Check sheet for the modelled part. Datum: model origin and axes. Units: mm. Coordinates: 2 decimals unless noted, no trailing zeros. Loops run counter-clockwise (first coordinate to the right, second up) from the corner with the lowest first, then second, coordinate; pieces in that order, holes last. Notation, with made-up numbers: M 42,-12.5 L 55,-12.5 A21 ccw 55,20.5 Z; hole C 52,-10.5 d1. An arc over 180 degrees is marked long. Answer as CSV lines item,"result". Start each with the question number.
from build123d import *

# Parameters (mm, degrees)
BASE_FLANGE1_DEPTH   = 3.03784
M8_CLEARANCE_HOLE1_D = 9


# Sheet-metal steps are written as plain solids
with BuildPart() as part:
    # Sketch1 → Base-Flange1 (new body)
    with BuildSketch(Plane(origin=(0, 0, 0), x_dir=(0, 0, -1), z_dir=(1, 0, 0))):
        with BuildLine():
            Line((-107.95, -152.4), (-222.25, -152.4))
            ThreePointArc((-222.25, -152.4), (-226.740128061, -150.540128061), (-228.6, -146.05))
            Line((-228.6, -146.05), (-228.6, 146.05))
            ThreePointArc((-228.6, 146.05), (-226.740128061, 150.540128061), (-222.25, 152.4))
            Line((-222.25, 152.4), (222.25, 152.4))
            ThreePointArc((222.25, 152.4), (226.740128061, 150.540128061), (228.6, 146.05))
            Line((228.6, 146.05), (228.6, -146.05))
            ThreePointArc((228.6, -146.05), (226.740128061, -150.540128061), (222.25, -152.4))
            Line((222.25, -152.4), (6.35, -152.4))
            ThreePointArc((6.35, -152.4), (1.859871939, -150.540128061), (0, -146.05))
            Line((0, -146.05), (0, -95.25))
            ThreePointArc((0, -95.25), (-1.859871939, -90.759871939), (-6.35, -88.9))
            Line((-6.35, -88.9), (-95.25, -88.9))
            ThreePointArc((-95.25, -88.9), (-99.740128061, -90.759871939), (-101.6, -95.25))
            Line((-101.6, -95.25), (-101.6, -146.05))
            ThreePointArc((-101.6, -146.05), (-103.459871939, -150.540128061), (-107.95, -152.4))
        make_face()
    extrude(amount=-BASE_FLANGE1_DEPTH)

    # M8 Clearance Hole1 (through all)
    with Locations(Plane(origin=(0, 0, 0), x_dir=(0, 0, -1), z_dir=(1, 0, 0))):
        with Locations((-209.55, 101.6), (-209.55, -101.6), (209.55, -101.6), (209.55, 101.6)):
            Hole(M8_CLEARANCE_HOLE1_D / 2)


solid = part.part
Item 1: Sectioned sample at B-B, the plane z = -209.55. Record the boundary of the cut face in (x, y), and give its area (3 significant figures).
Item 2: Sectioned sample at A-A, the plane y = 101.6. Record the boundary of the cut face in (x, z), and give its area (3 significant figures).
Item 3: Sectioned sample at D-D, the plane z = 88. Record the boundary of the cut face in (x, y).
Item 4: Release check for a two-part mould opening along Y. For faces 1 (the face through (-1.54, 99.88, -205.39)), 2 (the face through (-3.038, 2, -3)) record: released by +Y, released by -Y, zero draft, split by the parting line, or undercut.
Item 5: Sectioned sample at C-C, the plane x = -2.2. Record the boundary of the cut face in (y, z).
Item 6: Go/stop test with a flat-tipped pin: pin 1 (7 mm diameter, centred on y = 101.6, z = 209.55, fed in from -X) (3 decimals). Record where the tip stops, or that it passes through.
Item 7: Material ranges on line 1 (Y direction, x = -2.4, z = -209.55); line 2 (Z direction, x = -1.4, y = -105); line 3 (Y direction, x = -2.8, z = 19.5), recorded low to high. Write a range as from..to.
Reply:
1,outline,"M -3.04,-152.4 L 0,-152.4 L 0,-106.1 L -3.04,-106.1 Z; M -3.04,-97.1 L 0,-97.1 L 0,97.1 L -3.04,97.1 Z; M -3.04,106.1 L 0,106.1 L 0,152.4 L -3.04,152.4 Z"
1,area,"871 mm²"
2,outline,"M -3.04,-228.6 L 0,-228.6 L 0,-214.05 L -3.04,-214.05 Z; M -3.04,-205.05 L 0,-205.05 L 0,205.05 L -3.04,205.05 Z; M -3.04,214.05 L 0,214.05 L 0,228.6 L -3.04,228.6 Z"
2,area,"1,330 mm²"
3,outline,"M -3.04,-88.9 L 0,-88.9 L 0,152.4 L -3.04,152.4 Z"
4,face 1,"undercut"
4,face 2,"zero draft"
5,outline,"M -152.4,-222.25 A6.35 ccw -146.05,-228.6 L 146.05,-228.6 A6.35 ccw 152.4,-222.25 L 152.4,222.25 A6.35 ccw 146.05,228.6 L -146.05,228.6 A6.35 ccw -152.4,222.25 L -152.4,107.95 A6.35 ccw -146.05,101.6 L -95.25,101.6 A6.35 cw -88.9,95.25 L -88.9,6.35 A6.35 cw -95.25,0 L -146.05,0 A6.35 ccw -152.4,-6.35 Z; hole C -101.6,-209.55 d9; hole C -101.6,209.55 d9; hole C 101.6,-209.55 d9; hole C 101.6,209.55 d9"
6,pin 1,"through"
7,line 1,"-152.4..-106.1, -97.1..97.1, 106.1..152.4"
7,line 2,"-228.6..-212.5, -206.6..0, 101.6..206.6, 212.5..228.6"
7,line 3,"-88.9..152.4"
